from build123d import *

# Parameters (mm, degrees)
F0_R     = 3.175
F1_DEPTH = 5.08


with BuildPart() as f1:
    # F0 (on Top) → F1 (new body)
    with BuildSketch(Plane.XY):
        Polygon((-196.7800016522, 116.4700038791), (-196.7814051471, 116.4700038791), (-202.7097940445, 116.4700038791), (-202.7097940445, 108.8500038791), (-202.7097940445, 101.2300038791), (-202.7097940445, -23.2299961209), (-196.7800016522, -23.2299961209), (20.8102059555, -23.2299961209), (20.8102059555, 116.4700038791), (15.3085948529, 116.4700038791), (-35.4914051471, 116.4700038791), (-39.3014051471, 116.4700038791), (-90.9497940445, 116.4700038791), (-187.4697940445, 116.4700038791), (-189.1614051471, 116.4700038791), (-195.0897940445, 116.4700038791), align=None)
        with Locations((-196.3344303894, -15.6099961209)):
            Circle(F0_R, mode=Mode.SUBTRACT)
        Polygon((-189.1614051471, -18.3182691255), (-189.1614051471, 111.2217308745), (-189.1583133745, 111.2217308745), (-39.3014051471, 111.2217308745), (-39.3014051471, -18.3182691255), align=None, mode=Mode.SUBTRACT)
        with Locations((14.4348423004, -15.6099961209)):
            Circle(F0_R, mode=Mode.SUBTRACT)
        Polygon((-25.1297818765, 23.5917308745), (-25.1297818765, 69.3117308745), (7.8902181235, 69.3117308745), (7.8902181235, 23.5917308745), (7.8902181235, 5.8117308745), (-4.8097818765, 5.8117308745), (-8.6197818765, 5.8117308745), (-12.4297818765, 5.8117308745), (-25.1297818765, 5.8117308745), align=None, mode=Mode.SUBTRACT)
        with Locations((-196.3344303894, 108.8500038791)):
            Circle(F0_R, mode=Mode.SUBTRACT)
        with Locations((14.4348423004, 108.8500038791)):
            Circle(F0_R, mode=Mode.SUBTRACT)
        Polygon((7.8902181235, 23.5917308745), (-25.1297818765, 23.5917308745), (-25.1297818765, 5.8117308745), (-12.4297818765, 5.8117308745), (-12.4297818765, 12.1617308745), (-4.8097818765, 12.1617308745), (-4.8097818765, 5.8117308745), (7.8902181235, 5.8117308745), align=None)
    extrude(amount=F1_DEPTH)


solid = f1.part
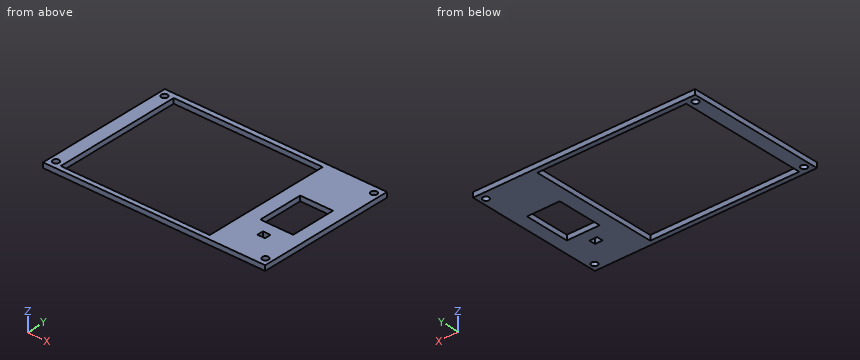
Build history of the part. All positions in model axes, mm. Round coordinates to 2 decimals unless told otherwise and drop trailing zeros. Write each loop counter-clockwise with the first axis right and the second up, starting at its lowest first coordinate (ties: lowest second). Pieces come first, ordered by that corner, then holes. Notation, with made-up numbers: M -18.5,20 L 31.5,20 A21 cw 31.5,51 Z; hole C 21.25,-7 d8. An arc over 180 degrees is marked long. Answer in a Markdown table with one row per item.
1. Saw through at B-B (y = 19.5). List the corners of the cut face in (x, z), and give its area (3 significant figures).
Geometry check:
| item | result |
|---|---|
| outline | M -202.71,0 L -189.16,0 L -189.16,5.08 L -202.71,5.08 Z; M -39.3,0 L 20.81,0 L 20.81,5.08 L -39.3,5.08 Z |
| area | 374 mm2 |
2. Saw through at C-C (z = 1.75). List the corners of the cut face in (x, y) (3 decimals).
Geometry check:
| item | result |
|---|---|
| outline | M -202.71,-23.23 L 20.81,-23.23 L 20.81,116.47 L -202.71,116.47 Z; hole C -196.334,-15.61 d6.35; hole C -196.334,108.85 d6.35; hole M -189.161,-18.318 L -39.301,-18.318 L -39.301,111.222 L -189.161,111.222 Z; hole M -25.13,23.592 L 7.89,23.592 L 7.89,69.312 L -25.13,69.312 Z; hole M -12.43,5.812 L -4.81,5.812 L -4.81,12.162 L -12.43,12.162 Z; hole C 14.435,-15.61 d6.35; hole C 14.435,108.85 d6.35 |
3. Probe L1, parallel to X at y = 25, z = 4.2; L2, parallel to Y at x = -61, z = 0.4; L3, parallel to X at y = 76.5, z = 1.75. List the from-to ranges inside material, lowest first. Write a range as [from, to].
Geometry check:
| item | result |
|---|---|
| L1 | [-202.71, -189.16], [-39.3, -25.13], [7.89, 20.81] |
| L2 | [-23.23, -18.32], [111.22, 116.47] |
| L3 | [-202.71, -189.16], [-39.3, 20.81] |
4. Saw through at A-A (x = 2.5). List the corners of the cut face in (y, z), and give its area (3 significant figures).
Geometry check:
| item | result |
|---|---|
| outline | M -23.23,0 L 23.59,0 L 23.59,5.08 L -23.23,5.08 Z; M 69.31,0 L 116.47,0 L 116.47,5.08 L 69.31,5.08 Z |
| area | 477 mm2 |
